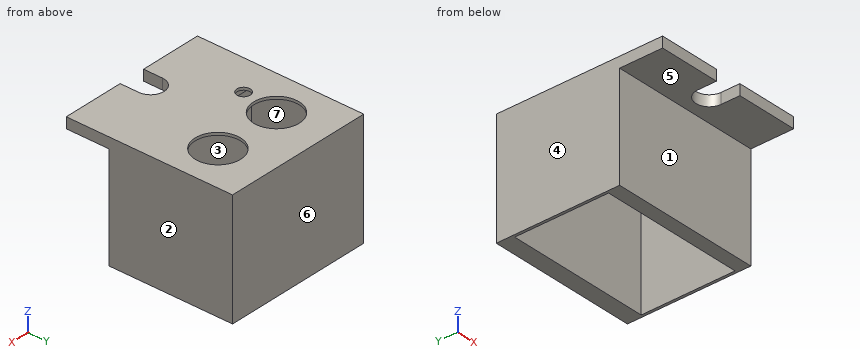
from build123d import *

# Parameters (mm, degrees)
SKETCH_R        = 8.5
SKETCH_R_2      = 2.5
PAD_DEPTH       = 43
SKETCH004_W     = 56
SKETCH004_H     = 16
SKETCH004_W_2   = 54
SKETCH004_H_2   = 35
POCKET_DEPTH    = 39
SKETCH006_W     = 54
SKETCH006_H     = 31
POCKET004_DEPTH = 3


with BuildPart() as part:
    # Sketch → Pad (new body)
    with BuildSketch(Plane.XY):
        with BuildLine():
            Line((56, 0), (56, 62))
            Line((56, 62), (0, 62))
            Line((0, 62), (0, 0))
            Line((0, 0), (23, 0))
            Line((23, 0), (23, 7))
            ThreePointArc((33, 7), (28, 12), (23, 7))
            Line((33, 0), (33, 7))
            Line((33, 0), (56, 0))
        make_face()
        with Locations((15.5, 43)):
            Circle(SKETCH_R, mode=Mode.SUBTRACT)
        with Locations((40.5, 43)):
            Circle(SKETCH_R, mode=Mode.SUBTRACT)
        with Locations((13.5, 29)):
            Circle(SKETCH_R_2, mode=Mode.SUBTRACT)
    extrude(amount=PAD_DEPTH)

    # Sketch004 (on Face12 of Pad) → Pocket (cut)
    with BuildSketch(Plane(origin=(0, 0, 0), x_dir=(1, 0, 0), z_dir=(0, 0, -1))):
        with Locations((28, -8)):
            Rectangle(SKETCH004_W, SKETCH004_H)
        with Locations((28, -38.5)):
            Rectangle(SKETCH004_W_2, SKETCH004_H_2)
    extrude(amount=-POCKET_DEPTH, mode=Mode.SUBTRACT)

    # Sketch006 (on Face20 of Pocket) → Pocket004 (cut)
    with BuildSketch(Plane(origin=(0, 0, 39), x_dir=(1, 0, 0), z_dir=(0, 0, -1))):
        with Locations((28, -40.5)):
            Rectangle(SKETCH006_W, SKETCH006_H)
    extrude(amount=-POCKET004_DEPTH, mode=Mode.SUBTRACT)


solid = part.part
The model under review builds one solid part; all positions refer to its coordinate system, in mm. Face numbers are marked on the shaded views. A direction names the side the tool comes from. Give positions to 0.01 mm unless a question says otherwise; leave off trailing zeros. Order: outer loops, then holes, each group sorted by start corner. A loop starts at its lowest first (then second) coordinate and runs counter-clockwise, first axis right, second up. Notation, with made-up numbers: M 59,-4 L 65,-4 A13 cw 65,21 Z; hole C -3.5,72 d11. An arc over 180 degrees is marked long. Use one line per item in the form item = value. Start each with the question number.
Item 1: Insertion check: pin 1 Ø15.5 at (x, y) = (20, 44.5) entering from -Z; pin 2 Ø2 at (x, z) = (27.5, 11.5) entering from -Y; pin 3 Ø5 at (x, y) = (41.5, 6.5) entering from -Z. Each pin has a flat end and moves straight along its axis. Give the tip position at first contact, or say it passes through.
Item 2: We need section D-D on x = 28. Give the boundary of the cut face in (y, z), plus the area to 3 significant figures.
Item 3: For the marked faces 5, 6 and 7, list the 3-axis set-ups (+Z, -Z, +X, -X, +Y, -Y) from which the entire face can be reached by the end or side of a thin tool; tool diameter is ignored.
Item 4: The part is to be moulded in two halves that separate along X. For the marked faces 1, 2, 3 and 4, say which applies: pulls with the +X half, pulls with the -X half, needs draft (parallel to the pull), parting line crosses it, or undercut.
Item 5: To check wall thickness, follow line 1 along Y through (x, z) = (14, 25); line 2 along X through (y, z) = (55.5, 20); line 3 along X through (y, z) = (29, 42.6). State the ranges of each line that lie inside material, in increasing order. Write a range as from..to.
Item 6: We need section C-C on z = 35. Give the boundary of the cut face in (x, y).
Item 7: We need section B-B on x = 40.5. Give the boundary of the cut face in (y, z), plus the area to 3 significant figures.
Item 8: We need section A-A on y = 5.5. Give the boundary of the cut face in (x, z), plus the area to 3 significant figures.
Completed:
q1.pin_1 = 42
q1.pin_2 = 16
q1.pin_3 = 39
q2.outline = M 12,39 L 16,39 L 16,0 L 21,0 L 21,39 L 25,39 L 25,42 L 56,42 L 56,0 L 62,0 L 62,43 L 12,43 Z
q2.area = 536 mm²
q3.face_5 = -Z, +X, -X, -Y
q3.face_6 = +Z, -Z, +X, -X, +Y
q3.face_7 = -Z
q4.face_1 = needs draft
q4.face_2 = pulls with the +X half
q4.face_3 = undercut
q4.face_4 = pulls with the -X half
q5.line_1 = 16..21, 56..62
q5.line_2 = 0..1, 55..56
q5.line_3 = 0..11, 16..56
q6.outline = M 0,16 L 56,16 L 56,62 L 0,62 Z; hole M 1,21 L 55,21 L 55,56 L 1,56 Z
q7.outline = M 0,39 L 16,39 L 16,0 L 21,0 L 21,39 L 25,39 L 25,42 L 34.5,42 L 34.5,43 L 0,43 Z; M 51.5,42 L 56,42 L 56,0 L 62,0 L 62,43 L 51.5,43 Z
q7.area = 567 mm²
q8.outline = M 0,39 L 23,39 L 23,43 L 0,43 Z; M 33,39 L 56,39 L 56,43 L 33,43 Z
q8.area = 184 mm²
